Check sheet for the modelled part. Datum: model origin and axes. Units: mm. Face numbers are marked on the shaded views. A direction names the side the tool comes from. Give positions to 0.01 mm unless a question says otherwise; leave off trailing zeros. Order: outer loops, then holes, each group sorted by start corner. A loop starts at its lowest first (then second) coordinate and runs counter-clockwise, first axis right, second up. Notation, with made-up numbers: M 77.5,60.5 L 93.5,60.5 A22 ccw 93.5,97.5 Z; hole C 56.5,-30 d2. An arc over 180 degrees is marked long. Return JSON: item names as keys, results as strings. Group by question number.
from build123d import *

# Parameters (mm, degrees)
PAD_DEPTH    = 12.7
SKETCH001_R  = 2.182812
POCKET_DEPTH = 27.433
CHAMFER_SIZE = 1


with BuildPart() as part:
    # Sketch → Pad (new body)
    with BuildSketch(Plane.XY):
        Polygon((0, -27.432), (15.24, -27.432), (15.24, -24.892), (2.54, -24.892), (2.54, 2.54), (-10.16, 2.54), (-10.16, 0), (0, 0), align=None)
    extrude(amount=PAD_DEPTH)

    # Sketch001 → Pocket (cut, through all)
    with BuildSketch(Plane.XZ):
        with Locations((8.89, 6.35)):
            Circle(SKETCH001_R)
        with Locations((-3.81, 6.35)):
            Circle(SKETCH001_R)
    extrude(amount=POCKET_DEPTH, mode=Mode.SUBTRACT)

    # Chamfer
    chamfer_edges = [part.edges().sort_by_distance(p)[0] for p in [
        (-10.16, 1.27, 0),
        (-10.16, 1.27, 12.7),
        (2.54, 2.54, 6.35),
        (15.24, -26.162, 0),
        (15.24, -26.162, 12.7),
    ]]
    chamfer(chamfer_edges, length=CHAMFER_SIZE)


solid = part.part
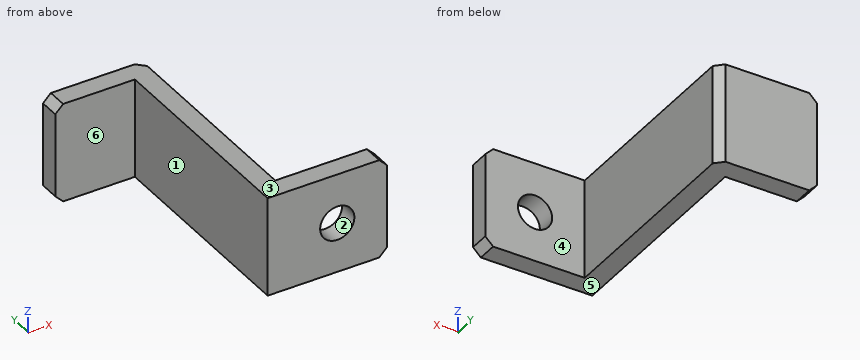
1) Tool access check on the marked faces 4, 5 and 6. Record the directions out of +Z, -Z, +X, -X, +Y, -Y that give a thin tool (end or side, any length) a straight path to the whole face; none if there is none.
2) Sectioned sample at A-A on x = 8.89. Record the boundary of the cut face in (y, z).
3) Sectioned sample at D-D on y = -3.25. Record the boundary of the cut face in (x, z).
4) Sectioned sample at C-C on z = 3. Record the boundary of the cut face in (x, y).
5) Release check for a two-part mould opening along X. For the marked faces 1, 2 and 3 record: released by +X, released by -X, zero draft, split by the parting line, or undercut.
6) Material ranges on line 1 along X through (y, z) = (-26.4, 6.35); line 2 along Z through (x, y) = (8.89, -26.7); line 3 along X through (y, z) = (-8.5, 9), recorded low to high.
7) Depth check by flat-ended pin: P1, Ø4, axis at y = -16, z = 6, coming from the +X side; P2, Ø1.5, axis at x = 3.5, z = 4.5, coming from the +Y side; P3, Ø2, axis at y = -22.5, z = 3, coming from the -X side. Enter the tip coordinate at first touch or a pass-through.
8) Sectioned sample at B-B on z = 6.35. Record the boundary of the cut face in (x, y).
Reply:
{
 "1": {"face 4": "+Z, -Z, +X, +Y", "face 5": "-Z, +X, -X, +Y, -Y", "face 6": "+Z, -Z, -X, -Y"},
 "2": {"outline": "M -27.43,0 L -24.89,0 L -24.89,4.17 L -27.43,4.17 Z; M -27.43,8.53 L -24.89,8.53 L -24.89,12.7 L -27.43,12.7 Z"},
 "3": {"outline": "M 0,0 L 2.54,0 L 2.54,12.7 L 0,12.7 Z"},
 "4": {"outline": "M -10.16,0 L 0,0 L 0,-27.43 L 15.24,-27.43 L 15.24,-24.89 L 2.54,-24.89 L 2.54,1.54 L 1.54,2.54 L -10.16,2.54 Z"},
 "5": {"face 1": "released by -X", "face 2": "undercut", "face 3": "zero draft"},
 "6": {"line 1": "0 to 6.71, 11.07 to 15.24", "line 2": "0 to 4.17, 8.53 to 12.7", "line 3": "0 to 2.54"},
 "7": {"P1": "x = 2.54", "P2": "y = -24.89", "P3": "x = 0"},
 "8": {"outline": "M -10.16,0 L 0,0 L 0,-27.43 L 6.71,-27.43 L 6.71,-24.89 L 2.54,-24.89 L 2.54,1.54 L 1.54,2.54 L -10.16,2.54 Z; M 11.07,-27.43 L 15.24,-27.43 L 15.24,-24.89 L 11.07,-24.89 Z"}
}
